Design review of the part shown in the three views and the two pictorial views. Dimensions are in mm from the part's minimum x, y and z. Round coordinates to 2 decimals unless told otherwise and drop trailing zeros. Loops run counter-clockwise (first coordinate to the right, second up) from the corner with the lowest first, then second, coordinate; pieces in that order, holes last. Notation, with made-up numbers: (-2.75, 17.5) -> (55.25, 17.5) arc R18 cw to (55.25, 41.5) -> close; hole circle Ø3 at (10.5, 58). An arc over 180 degrees is marked (long way). Use a Markdown table: item, result. Add a question column.
1) Consider section C-C on y = 8. Give the boundary of the cut face in (x, z).
2) Wall thickness on probe 1 along Y at (x, z) = (0.85, 25); probe 2 along Z at (x, y) = (1.7, 112); probe 3 along Z at (x, y) = (0.7, 8): over which ranges is each line inside the solid? List them lowest first.
3) Consider section B-B on z = 146. Give the boundary of the cut face in (x, y).
4) Consider section A-A on y = 112. Give the boundary of the cut face in (x, z), plus the area to 4 significant figures.
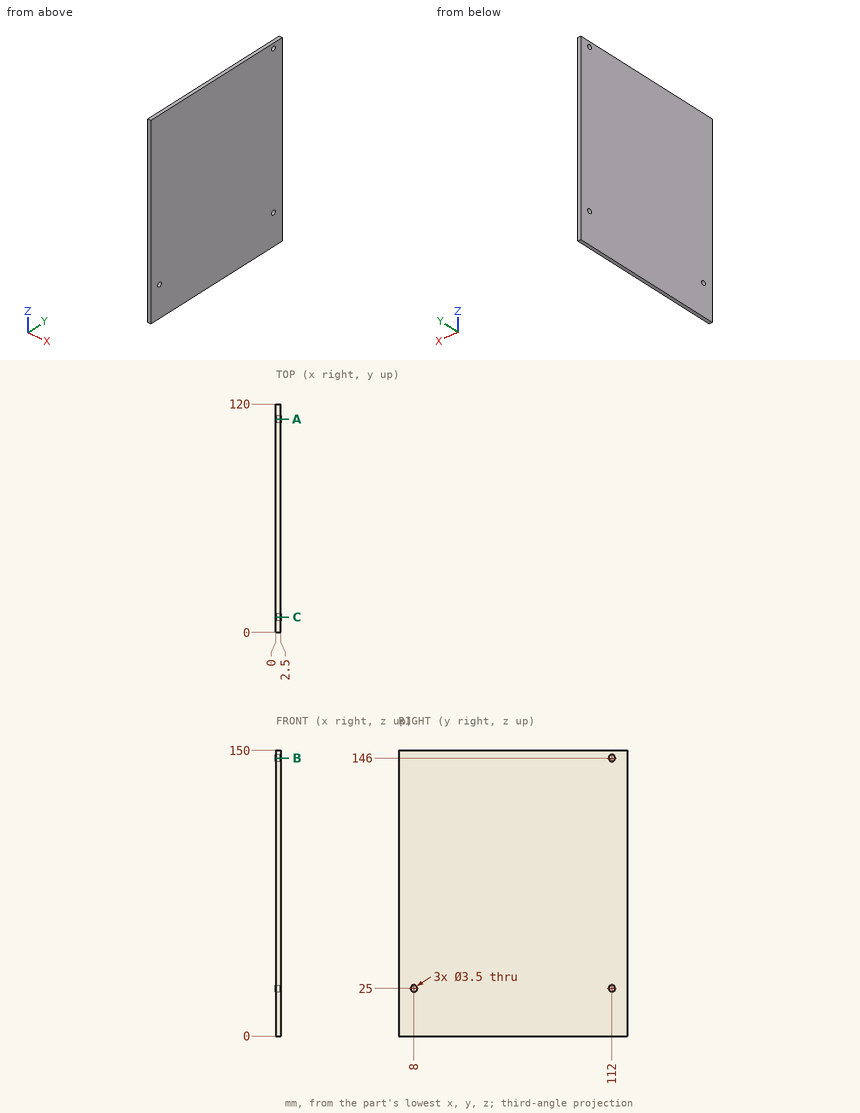
Result set:
| question | item | result |
|---|---|---|
| 1 | outline | (0, 0) -> (2.5, 0) -> (2.5, 23.25) -> (0, 23.25) -> close; (0, 26.75) -> (2.5, 26.75) -> (2.5, 150) -> (0, 150) -> close |
| 2 | probe 1 | 0 to 6.25, 9.75 to 110.25, 113.75 to 120 |
| 2 | probe 2 | 0 to 23.25, 26.75 to 144.25, 147.75 to 150 |
| 2 | probe 3 | 0 to 23.25, 26.75 to 150 |
| 3 | outline | (0, 0) -> (2.5, 0) -> (2.5, 110.25) -> (0, 110.25) -> close; (0, 113.75) -> (2.5, 113.75) -> (2.5, 120) -> (0, 120) -> close |
| 4 | outline | (0, 0) -> (2.5, 0) -> (2.5, 23.25) -> (0, 23.25) -> close; (0, 26.75) -> (2.5, 26.75) -> (2.5, 144.25) -> (0, 144.25) -> close; (0, 147.75) -> (2.5, 147.75) -> (2.5, 150) -> (0, 150) -> close |
| 4 | area | 357.5 mm2 |
